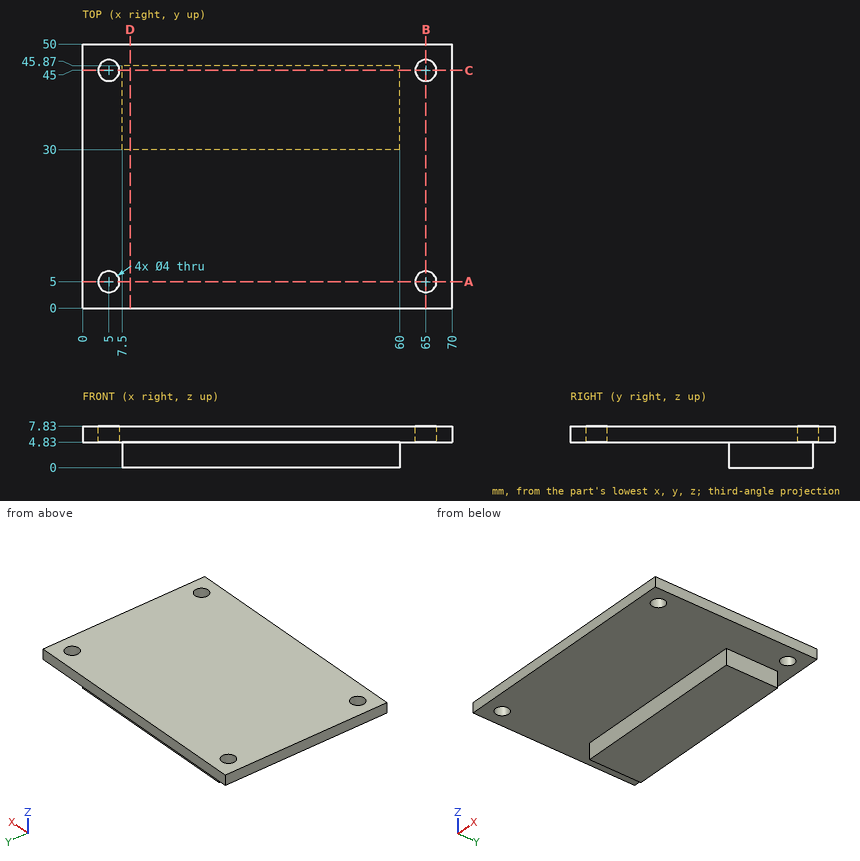
Geometry check sheet. Reference: drawing and pictorial views, mm from the part's lowest x, y, z. Give positions to 0.01 mm unless a question says otherwise; leave off trailing zeros. Write each loop counter-clockwise with the first axis right and the second up, starting at its lowest first coordinate (ties: lowest second). Pieces come first, ordered by that corner, then holes. Notation, with made-up numbers: (73.25, 64) - (97.25, 64) arc R19 ccw to (97.25, 80) - close; hole circle Ø11 at (76.25, 54). An arc over 180 degrees is marked (long way). Put each result on its own line as item: value.
Q1. Section check B-B on x = 65. Record the cut outline in (y, z), and give its area (3 significant figures).
Result:
outline: (0, 4.83) - (3, 4.83) - (3, 7.83) - (0, 7.83) - close; (7, 4.83) - (43, 4.83) - (43, 7.83) - (7, 7.83) - close; (47, 4.83) - (50, 4.83) - (50, 7.83) - (47, 7.83) - close
area: 126 mm2
Q2. Section check A-A on y = 5. Record the cut outline in (x, z), and give its area (3 significant figures).
Result:
outline: (0, 4.83) - (3, 4.83) - (3, 7.83) - (0, 7.83) - close; (7, 4.83) - (63, 4.83) - (63, 7.83) - (7, 7.83) - close; (67, 4.83) - (70, 4.83) - (70, 7.83) - (67, 7.83) - close
area: 186 mm2
Q3. Depth check by flat-ended pin: P1, Ø1.5, axis at x = 16, z = 2, coming from the +Y side; P2, Ø3.5, axis at x = 5, y = 45, coming from the -Z side; P3, Ø6.5, axis at x = 65, y = 45, coming from the -Z side; P4, Ø4, axis at y = 39, z = 1.5, coming from the -X side. Enter the tip coordinate at first touch or a pass-through.
Result:
P1: y = 45.87
P2: through
P3: z = 4.83
P4: x = 7.5
Q4. Scan lines: probe 1 along Y at (x, z) = (65, 6.05); probe 2 along Z at (x, y) = (53.5, 22.5); probe 3 along Y at (x, z) = (13.5, 3.25). Record each from-to range of solid material in increasing order. Write a range as from..to.
Result:
probe 1: 0..3, 7..43, 47..50
probe 2: 4.83..7.83
probe 3: 30..45.87
Q5. Section check C-C on y = 45. Record the cut outline in (x, z).
Result:
outline: (0, 4.83) - (3, 4.83) - (3, 7.83) - (0, 7.83) - close; (7, 4.83) - (7.5, 4.83) - (7.5, 0) - (60, 0) - (60, 4.83) - (63, 4.83) - (63, 7.83) - (7, 7.83) - close; (67, 4.83) - (70, 4.83) - (70, 7.83) - (67, 7.83) - close
Q6. Section check D-D on x = 9. Record the cut outline in (y, z), and give its area (3 significant figures).
Result:
outline: (0, 4.83) - (30, 4.83) - (30, 0) - (45.87, 0) - (45.87, 4.83) - (50, 4.83) - (50, 7.83) - (0, 7.83) - close
area: 227 mm2
